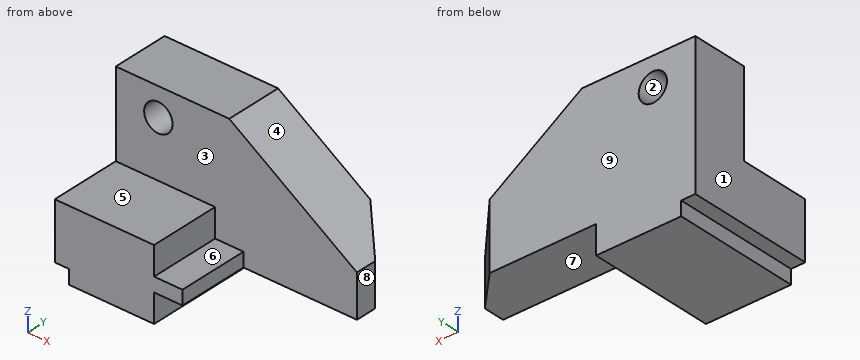
from build123d import *

# Parameters (mm, degrees)
F1_DEPTH      = 25.4
F3_DEPTH      = 25.4
F3_DEPTH_BACK = 31.75
F4_DEPTH      = 31.75
F5_R          = 6.35
F6_DEPTH      = 25.401
F8_DEPTH      = 57.151


with BuildPart() as f1:
    # F0 (on Front) → F1 (new body)
    with BuildSketch(Plane.XZ):
        Polygon((0, 57.15), (0, 0), (107.95, 0), (107.95, 19.05), (50.8, 57.15), align=None)
    extrude(amount=F1_DEPTH)

    # F2 (on face) → F3 (join, two sides)
    with BuildSketch(Plane.XZ.offset(25.4)) as f3_sk:
        Polygon((44.45, 0), (0, 0), (0, -6.35), (6.35, -6.35), (6.35, -12.7), (44.45, -12.7), align=None)
    extrude(amount=-F3_DEPTH)
    extrude(f3_sk.sketch, amount=F3_DEPTH_BACK)

    # F2 (on face) → F4 (join)
    with BuildSketch(Plane.XZ.offset(25.4)):
        Polygon((0, 19.05), (0, 0), (44.45, 0), (57.15, 0), (57.15, 6.35), (44.45, 6.35), (44.45, 19.05), align=None)
    extrude(amount=F4_DEPTH)

    # F5 (on face) → F6 (cut, through all)
    with BuildSketch(Plane.XZ.offset(25.4)):
        with Locations((19.05, 44.45)):
            Circle(F5_R)
    extrude(amount=-F6_DEPTH, mode=Mode.SUBTRACT)

    # F7 (on face) → F8 (cut, through all)
    with BuildSketch(Plane(origin=(0, 0, 0), x_dir=(1, 0, 0), z_dir=(0, 0, -1))):
        Polygon((107.95, 0), (107.95, 15.875), (92.075, 0), align=None)
    extrude(amount=-F8_DEPTH, mode=Mode.SUBTRACT)


solid = f1.part
The listing builds one solid part. Answer for the finished solid, in the listing's coordinates (mm). Face numbers are marked on the shaded views. A direction names the side the tool comes from. Give positions to 0.01 mm unless a question says otherwise; leave off trailing zeros. Write each loop counter-clockwise with the first axis right and the second up, starting at its lowest first coordinate (ties: lowest second). Pieces come first, ordered by that corner, then holes.
Item 1: Section C-C, the plane y = -20 is taken. Write down the section's boundary in (x, z), plus the area to 3 significant figures.
Item 2: Which of the six approach directions +Z, -Z, +X, -X, +Y, -Y give full straight-line access (tool end or side, diameter ignored) to the marked faces 5, 6, 7, 8 and 9?
Item 3: Section B-B, the plane z = 44.45 is taken. Write down the section's boundary in (x, y), plus the area to 3 significant figures.
Item 4: Determine the mould class of the marked faces 1, 2, 3 and 4 for opening direction X: released by +X, released by -X, zero draft, split by the parting line, or undercut.
Item 5: Find the intervals of material crossed by line 1 along Z through (x, y) = (19.05, -16.5); line 2 along Z through (x, y) = (28.5, -41.5); line 3 along Y through (x, z) = (7, 19.5), in increasing order.
Item 6: Section A-A, the plane x = 19.05 is taken. Write down the section's boundary in (y, z), plus the area to 3 significant figures.
Item 7: Section D-D, the plane x = 31 is taken. Write down the section's boundary in (y, z).
Item 8: Flat-ended cylindrical pins translate along their axes: P1, Ø6.5, axis at y = -27, z = -7.5, coming from the +X side; P2, Ø5, axis at x = 61.5, z = 37, coming from the -Y side; P3, Ø1.9, axis at y = -40.5, z = 4, coming from the +X side. Find the tip coordinate at first contact, or state that the pin passes through.
Completed:
1. outline: (0, -6.35) - (6.35, -6.35) - (6.35, -12.7) - (44.45, -12.7) - (44.45, 0) - (107.95, 0) - (107.95, 19.05) - (50.8, 57.15) - (0, 57.15) - close; hole circle Ø12.7 at (19.05, 44.45)
1. area: 5,480 mm2
2. face 5: +Z, +X, -X, -Y
2. face 6: +Z, +X, -Y
2. face 7: -Z, +X, +Y, -Y
2. face 8: +Z, -Z, +X, +Y, -Y
2. face 9: +Z, -Z, +X, -X, +Y
3. outline: (0, -25.4) - (12.7, -25.4) - (12.7, 0) - (0, 0) - close; (25.4, -25.4) - (69.85, -25.4) - (69.85, 0) - (25.4, 0) - close
3. area: 1,450 mm2
4. face 1: released by -X
4. face 2: undercut
4. face 3: zero draft
4. face 4: released by +X
5. line 1: z = -12.7 to 38.1, 50.8 to 57.15
5. line 2: z = -12.7 to 19.05
5. line 3: y = -25.4 to 0
6. outline: (-57.15, -12.7) - (0, -12.7) - (0, 38.1) - (-25.4, 38.1) - (-25.4, 19.05) - (-57.15, 19.05) - close; (-25.4, 50.8) - (0, 50.8) - (0, 57.15) - (-25.4, 57.15) - close
6. area: 2,460 mm2
7. outline: (-57.15, -12.7) - (0, -12.7) - (0, 57.15) - (-25.4, 57.15) - (-25.4, 19.05) - (-57.15, 19.05) - close
8. P1: stops at x = 44.45
8. P2: stops at y = -25.4
8. P3: stops at x = 57.15
